```python
from build123d import *

# Parameters (mm, degrees)
SKETCH033_W     = 30
SKETCH033_H     = 32
PAD023_DEPTH    = 6
PAD024_DEPTH    = 6
SKETCH035_R     = 1.575
POCKET011_DEPTH = 6
SKETCH045_W     = 20
SKETCH045_H     = 6
PAD030_DEPTH    = 20
POCKET016_DEPTH = 12
SKETCH047_R     = 1.6
POCKET017_DEPTH = 6
SKETCH048_R     = 3
POCKET018_DEPTH = 2.5
SKETCH049_R     = 3
POCKET019_DEPTH = 2.5
SKETCH084_W     = 4
SKETCH084_H     = 6
PAD049_DEPTH    = 14
SKETCH085_R     = 3.975
POCKET036_DEPTH = 5.2


with BuildPart() as part:
    # Sketch033 → Pad023 (new body)
    with BuildSketch(Plane.XZ):
        Rectangle(SKETCH033_W, SKETCH033_H)
    extrude(amount=PAD023_DEPTH)

    # Sketch034 (on Face6 of Pad023) → Pad024 (join)
    with BuildSketch(Plane.XZ.offset(6)):
        Polygon((-15, 16), (15, 16), (27, 16), (27, -16), (15, -16), (-15, -16), (-27, -16), (-27, 0), (-37, 16), (-37, 32), (-17, 32), (-17, 16), align=None)
    extrude(amount=-PAD024_DEPTH)

    # Sketch035 (on Face9 of Pad024) → Pocket011 (cut)
    with BuildSketch(Plane.XZ.offset(6)):
        with Locations((-10, 10)):
            Circle(SKETCH035_R)
        with Locations((10, 10)):
            Circle(SKETCH035_R)
        with Locations((10, -10)):
            Circle(SKETCH035_R)
        with Locations((-10, -10)):
            Circle(SKETCH035_R)
    extrude(amount=-POCKET011_DEPTH, mode=Mode.SUBTRACT)

    # Sketch045 → Pad030 (join)
    with BuildSketch(Plane(origin=(0, 0, 0), x_dir=(1, 0, 0), z_dir=(0, 1, 0))):
        with Locations((-27, -19)):
            Rectangle(SKETCH045_W, SKETCH045_H)
    extrude(amount=PAD030_DEPTH)

    # Sketch046 (on Face13 of Pad030) → Pocket016 (cut)
    with BuildSketch(Plane(origin=(0, 0, 16), x_dir=(1, 0, 0), z_dir=(0, 0, -1))):
        with BuildLine():
            ThreePointArc((-21.05, -10), (-27, -4.05), (-32.95, -10))
            Line((-32.95, -10), (-32.95, -25))
            ThreePointArc((-32.95, -25), (-27, -30.95), (-21.05, -25))
            Line((-21.05, -10), (-21.05, -25))
        make_face()
    extrude(amount=-POCKET016_DEPTH, mode=Mode.SUBTRACT)

    # Sketch047 (on Face4 of Pocket016) → Pocket017 (cut)
    with BuildSketch(Plane.XZ.offset(6)):
        with Locations((10, -4)):
            Circle(SKETCH047_R)
        with Locations((10, 4)):
            Circle(SKETCH047_R)
        with Locations((-10, 0)):
            Circle(SKETCH047_R)
    extrude(amount=-POCKET017_DEPTH, mode=Mode.SUBTRACT)

    # Sketch048 (on Face4 of Pocket017) → Pocket018 (cut)
    with BuildSketch(Plane.XZ.offset(6)):
        with Locations((-10, 10)):
            Circle(SKETCH048_R)
        with Locations((10, 10)):
            Circle(SKETCH048_R)
        with Locations((10, -10)):
            Circle(SKETCH048_R)
        with Locations((-10, -10)):
            Circle(SKETCH048_R)
    extrude(amount=-POCKET018_DEPTH, mode=Mode.SUBTRACT)

    # Sketch049 (on Face5 of Pocket018) → Pocket019 (cut)
    with BuildSketch(Plane(origin=(0, 0, 0), x_dir=(1, 0, 0), z_dir=(0, 1, 0))):
        with Locations((-10, 0)):
            Circle(SKETCH049_R)
        with Locations((10, 4)):
            Circle(SKETCH049_R)
        with Locations((10, -4)):
            Circle(SKETCH049_R)
    extrude(amount=-POCKET019_DEPTH, mode=Mode.SUBTRACT)

    # Sketch084 (on Face8 of Pad024) → Pad049 (join)
    with BuildSketch(Plane(origin=(0, 0, 0), x_dir=(1, 0, 0), z_dir=(0, 1, 0))):
        with Locations((19, 13)):
            Rectangle(SKETCH084_W, SKETCH084_H)
    extrude(amount=PAD049_DEPTH)

    # Sketch085 (on Face4 of Pad049) → Pocket036 (cut)
    with BuildSketch(Plane(origin=(0, 0, 0), x_dir=(1, 0, 0), z_dir=(0, 1, 0))):
        with Locations((21, 0)):
            Circle(SKETCH085_R)
        with Locations((-21, 7)):
            Circle(SKETCH085_R)
        with Locations((-21, -7)):
            Circle(SKETCH085_R)
    extrude(amount=-POCKET036_DEPTH, mode=Mode.SUBTRACT)


with BuildPart() as part_1:
    # Body005 placement: moved
    add(part.part.moved(Location((-1, -37, 39.4))))


solid = part_1.part
```
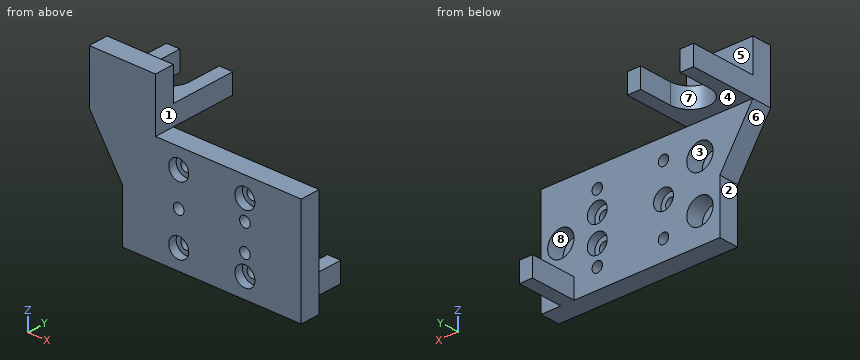
Here's how the part is built. I have some questions about the finished solid (model axes, mm). Face numbers are marked on the shaded views. A direction names the side the tool comes from. Give positions to 0.01 mm unless a question says otherwise; leave off trailing zeros. Loops run counter-clockwise (first coordinate to the right, second up) from the corner with the lowest first, then second, coordinate; pieces in that order, holes last. Notation, with made-up numbers: (79.5, 4.5) -> (116.5, 4.5) arc R11 cw to (116.5, 24.5) -> close; hole circle Ø3 at (-25.75, -22.75). An arc over 180 degrees is marked (long way). Use one line per item in the form item = value. Start each with the question number.
1) Imagine slicing it at D-D (z = 54). Please give me the cut outline in (x, y) (3 decimals).
2) Which directions (+Z, -Z, +X, -X, +Y, -Y) give clear straight access to the entire face, cutting with the end or side of a thin tool? Please do the marked faces 1, 2, 3 and 4.
3) Imagine slicing it at C-C (x = 9). Count the separate pieces of the cut face and the enclosed holes in it, then the cut area to 4 significant figures.
4) Imagine slicing it at A-A (y = -32). Please give me the cut outline in (x, z), then the cut area to 3 significant figures.
5) Please list where these lines run through material, in increasing order: line 1 along Z through (x, y) = (-11, -41.7); line 2 along X through (y, z) = (-38, 39.4) (3 decimals); line 3 along Z through (x, y) = (9, -38.2) (3 decimals).
6) Thinking about a two-plate mould opening in X: for the marked faces 5, 6, 7 and 8, which applies, +X half, -X half, draft (parallel to the pull), parting line (faces both ways), or undercut?
7) For P1, Ø9.5, axis at x = 9, z = 43.4, coming from the -Y side; P2, Ø6, axis at y = -28.5, z = 60.5, coming from the +X side; P3, Ø3.5, axis at x = 9, z = 35.4, coming from the +Y side; P4, Ø3, axis at x = 17, y = -30, coming from the +Z side, each with a flat end and sliding along its axis, tell me the tip position at first contact or that it passes through.
8) Imagine slicing it at B-B (x = 21). Please give me the cut outline in (y, z).
Check values:
q1.outline = (-37.125, -43) -> (26, -43) -> (26, -37) -> (-37.125, -37) -> close
q2.face_1 = +Z, +X, +Y, -Y
q2.face_2 = -Z, -X, +Y, -Y
q2.face_3 = +Y
q2.face_4 = -Z, +X, -X, +Y
q3.separate_pieces = 5
q3.enclosed_holes = 0
q3.area = 87.55 mm^2
q4.outline = (-38, 55.4) -> (-31.23, 55.4) -> (-31.23, 61.4) -> (-38, 61.4) -> close; (-24.77, 55.4) -> (-18, 55.4) -> (-18, 61.4) -> (-24.77, 61.4) -> close; (16, 23.4) -> (20, 23.4) -> (20, 29.4) -> (16, 29.4) -> close
q4.area = 105 mm^2
q5.line_1 = 23.4 to 26.4, 32.4 to 37.8, 41 to 46.4, 52.4 to 55.4
q5.line_2 = -28 to -14, -8 to 16.025, 23.975 to 26
q5.line_3 = 23.4 to 27.825, 30.975 to 32.4, 38.4 to 40.4, 46.4 to 47.825, 50.975 to 55.4
q6.face_5 = draft
q6.face_6 = -X half
q6.face_7 = undercut
q6.face_8 = undercut
q7.P1 = -43
q7.P2 = -18
q7.P3 = -39.5
q7.P4 = 29.4
q8.outline = (-43, 23.4) -> (-37, 23.4) -> (-37, 35.55) -> (-42.2, 35.55) -> (-42.2, 43.25) -> (-37, 43.25) -> (-37, 55.4) -> (-43, 55.4) -> close
